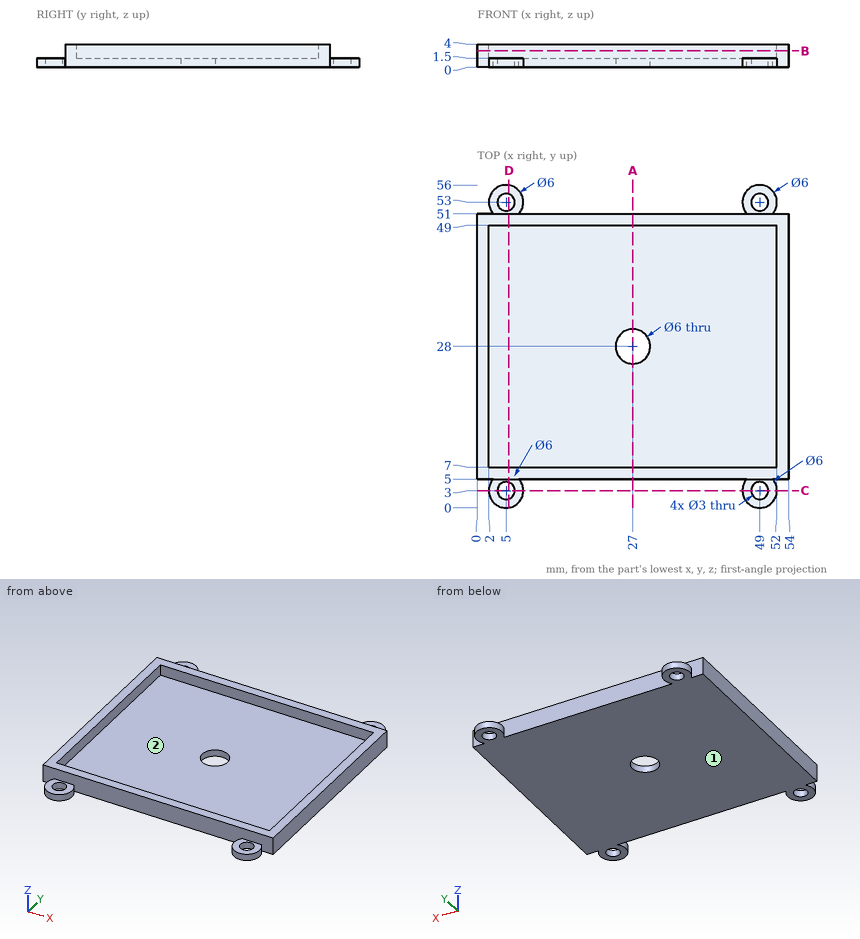
Could you check a few things on this drawing? It's one solid part, dimensions in mm from its lowest x, y, z. Round coordinates to 2 decimals unless told otherwise and drop trailing zeros. Write each loop counter-clockwise with the first axis right and the second up, starting at its lowest first coordinate (ties: lowest second). Pieces come first, ordered by that corner, then holes. Notation, with made-up numbers: (28.5, 24) -> (84.5, 24) arc R11 cw to (84.5, 43) -> close; hole circle Ø6 at (58.5, 77.5). An arc over 180 degrees is marked (long way). Use one line per item in the form item = value. Start each with the question number.
Q1. If I drill on probe 1 along X at (y, z) = (29, 3); probe 2 along Y at (x, z) = (27, 0.85); probe 3 along Y at (x, z) = (33.5, 3.55), over which ranges is the centre line in solid material (lowest first)? Write a range as [from, to].
Q2. I'm going to push flat-ended pins straight in: P1, Ø1.8, axis at x = 5, y = 3, coming from the +Z side; P2, Ø2, axis at x = 35.5, z = 2.5, coming from the -Y side; P3, Ø1.2, axis at x = 21, z = 2, coming from the +Y side; P4, Ø1.5, axis at x = 50, y = 1.5, coming from the +Z side. Where does each tip first touch, or does it pass through?
Q3. Imagine slicing it at B-B (z = 2.8). Please give me the cut outline in (x, y), then the cut area to 3 significant figures.
Q4. We'd pull the mould along Y, two halves only. Please class the marked faces 1 and 2: +Y half, -Y half, draft (parallel to the pull), parting line (faces both ways), or undercut.
Q5. Imagine slicing it at A-A (x = 27). Please give me the cut outline in (y, z), then the cut area to 3 significant figures.
Q6. Imagine slicing it at D-D (x = 5.5). Please give me the cut outline in (y, z), then the cut area to 3 significant figures.
Q7. Imagine slicing it at C-C (y = 3). Please give me the cut outline in (x, z), then the cut area to 3 significant figures.
Worked out:
q1.probe_1 = [0, 2], [52, 54]
q1.probe_2 = [5, 25], [31, 51]
q1.probe_3 = [5, 7], [49, 51]
q2.P1 = through
q2.P2 = 5
q2.P3 = 51
q2.P4 = 1.5
q3.outline = (0, 5) -> (54, 5) -> (54, 51) -> (0, 51) -> close; hole (2, 7) -> (52, 7) -> (52, 49) -> (2, 49) -> close
q3.area = 384 mm^2
q4.face_1 = draft
q4.face_2 = undercut
q5.outline = (5, 0) -> (25, 0) -> (25, 1.5) -> (7, 1.5) -> (7, 4) -> (5, 4) -> close; (31, 0) -> (51, 0) -> (51, 4) -> (49, 4) -> (49, 1.5) -> (31, 1.5) -> close
q5.area = 70.0 mm^2
q6.outline = (0.04, 0) -> (1.59, 0) -> (1.59, 1.5) -> (0.04, 1.5) -> close; (4.41, 0) -> (51.59, 0) -> (51.59, 1.5) -> (51, 1.5) -> (51, 4) -> (49, 4) -> (49, 1.5) -> (7, 1.5) -> (7, 4) -> (5, 4) -> (5, 1.5) -> (4.41, 1.5) -> close; (54.41, 0) -> (55.96, 0) -> (55.96, 1.5) -> (54.41, 1.5) -> close
q6.area = 85.4 mm^2
q7.outline = (2, 0) -> (3.5, 0) -> (3.5, 1.5) -> (2, 1.5) -> close; (6.5, 0) -> (8, 0) -> (8, 1.5) -> (6.5, 1.5) -> close; (46, 0) -> (47.5, 0) -> (47.5, 1.5) -> (46, 1.5) -> close; (50.5, 0) -> (52, 0) -> (52, 1.5) -> (50.5, 1.5) -> close
q7.area = 9.00 mm^2
